```python
from build123d import *

# Parameters (mm, degrees)
F0_R      = 6.35
F1_DEPTH  = 0.254
F2_R      = 3.429
F3_DEPTH  = 1.905
F3_TAPER  = 20
F4_T      = 0.254
F5_R      = 1.0795
F6_DEPTH  = 25.4
F7_R      = 0.3175
F8_DEPTH  = 25.4
F9_R      = 0.3175
F10_DEPTH = 25.4


# Not quite as in the source:
# - a shell that OpenCascade refuses in one call is made with other operations: the cavity is built on its own and cut out


with BuildPart() as f1:
    # F0 (on Top) → F1 (new body)
    with BuildSketch(Plane.XY):
        Circle(F0_R)
    extrude(amount=F1_DEPTH)

    # F2 (on face) → F3 (join)
    with BuildSketch(Plane.XY.offset(0.254)):
        Circle(F2_R)
    extrude(amount=F3_DEPTH, taper=F3_TAPER)

    # F4: shell of thickness 0.254, made by hand


with BuildPart() as f4_core1:
    # F4_t2: copy of F1
    add(f1.part)

    # the walls: a layer under each face that stays
    f4_faces = [f4_core1.faces().sort_by_distance(p)[0] for p in [
        (-6.35, 0, 0.127),
        (-4.2333333333, -4.2333333333, 0.254),
        (-3.0823183519, 0, 1.2065),
        (0, 0, 2.159),
    ]]
    thicken(f4_faces, amount=-F4_T, mode=Mode.SUBTRACT)

    # F4_s3 → F4_t4 (revolve, cut)
    with BuildSketch(Plane.XZ):
        Polygon((3.4313868193, 0.2574087312), (3.429, 0), (3.2511472853, 0), (3.1903180743, 0.1671268836), align=None)
    revolve(axis=Axis((0, 0, 0.254), (0, 0, -1)), mode=Mode.SUBTRACT)


with BuildPart() as f1_1:
    add(f1.part)

    # what is left inside the walls is the cavity
    f4_cavity = [f4_core1.part.solids().sort_by_distance(p)[0] for p in [
        (-2.977087, 0, 0.745549),
    ]]
    add(f4_cavity, mode=Mode.SUBTRACT)

    # F5 (on face) → F6 (cut)
    with BuildSketch(Plane.XY.offset(2.159)):
        Circle(F5_R)
    extrude(amount=-F6_DEPTH, mode=Mode.SUBTRACT)

    # F7 (on face) → F8 (cut)
    with BuildSketch(Plane.XY.offset(2.159)):
        with Locations((-1.3804862777, 1.0167437666)):
            Circle(F7_R)
        with Locations((-1.5707690699, -0.6871643028)):
            Circle(F7_R)
        with Locations((-0.1902827922, -1.7039080694)):
            Circle(F7_R)
        with Locations((1.3804862777, -1.0167437666)):
            Circle(F7_R)
        with Locations((1.5707690699, 0.6871643028)):
            Circle(F7_R)
        with Locations((0.1902827922, 1.7039080694)):
            Circle(F7_R)
    extrude(amount=-F8_DEPTH, mode=Mode.SUBTRACT)

    # F9 (on face) → F10 (cut)
    with BuildSketch(Plane.XY.offset(0.254)):
        with Locations((-3.3923081987, 4.5992901719)):
            Circle(F9_R)
        with Locations((-5.1411364532, 2.4959849698)):
            Circle(F9_R)
        with Locations((-5.7121923037, -0.179120309)):
            Circle(F9_R)
        with Locations((-4.9746537368, -2.8131912837)):
            Circle(F9_R)
        with Locations((-3.0974819499, -4.8027940378)):
            Circle(F9_R)
        with Locations((-0.510714377, -5.6921345579)):
            Circle(F9_R)
        with Locations((2.193051705, -5.2774756484)):
            Circle(F9_R)
        with Locations((4.3944160704, -3.6538106683)):
            Circle(F9_R)
        with Locations((5.5890726726, -1.1931016973)):
            Circle(F9_R)
        with Locations((5.5033400811, 1.5409324941)):
            Circle(F9_R)
        with Locations((4.1568585995, 3.9219576214)):
            Circle(F9_R)
        with Locations((1.8580909083, 5.4045095223)):
            Circle(F9_R)
        with Locations((-0.8663430176, 5.6489534231)):
            Circle(F9_R)
    extrude(amount=-F10_DEPTH, mode=Mode.SUBTRACT)


solid = f1_1.part
```
Source: CAD feature listing. Evaluate the final solid. Frame: model axes, mm. A direction names the side the tool comes from. Give positions to 0.01 mm unless a question says otherwise; leave off trailing zeros. Order: outer loops, then holes, each group sorted by start corner. A loop starts at its lowest first (then second) coordinate and runs counter-clockwise, first axis right, second up. Notation, with made-up numbers: (-10, -19) -> (0, -19) arc R20 ccw to (0, -12) -> close; hole circle Ø3 at (-9.75, -4.75). An arc over 180 degrees is marked (long way). Use a Markdown table: item, result.
Q1. Section A-A (z = 0.8). Return the cut outline in (x, y), and give its area (3 significant figures).
A:
| item | result |
|---|---|
| outline | circle Ø6.46 at (0, 0); hole circle Ø5.92 at (0, 0) |
| area | 5.26 mm^2 |
Q2. First-contact query: P1, Ø1, axis at x = -1.5, z = 2, coming from the +Y side; P2, Ø1, axis at x = -2, y = -4.5, coming from the +Z side; P3, Ø4, axis at x = 1, y = 1, coming from the -Z side; P4, Ø2.5, axis at x = 0, y = 0, coming from the -Z side (3 decimals). Flat tips, straight axial feed; report the tip coordinate or a pass-through.
A:
| item | result |
|---|---|
| P1 | y = 2.69 |
| P2 | z = 0.25 |
| P3 | z = 0 |
| P4 | z = 1.905 |
Q3. Section B-B (x = -4.25). Return the cut outline in (y, z).
A:
| item | result |
|---|---|
| outline | (-4.72, 0) -> (4.72, 0) -> (4.72, 0.25) -> (-4.72, 0.25) -> close |
Q4. Access query for faces 1 (the face through (3, -3, 0.254)), 2 (the face through (-3, 2, 0)). Directions: +Z, -Z, +X, -X, +Y, -Y. A direction counts if a zero-diameter tool reaches every point of the face in a straight line with its end or side. Return the directions, or none.
A:
| item | result |
|---|---|
| face 1 | +Z |
| face 2 | -Z, +X, -X, +Y, -Y |
Q5. Section C-C (z = 1.6). Return the cut outline in (x, y).
A:
| item | result |
|---|---|
| outline | circle Ø5.88 at (0, 0); hole circle Ø5.34 at (0, 0) |
Q6. Material intervals for line 1 (X direction, y = 1.75, z = 0.1); line 2 (Y direction, x = -1, z = 0.3); line 3 (X direction, y = 0, z = 0.85), sorted ascending. Write a range as [from, to].
A:
| item | result |
|---|---|
| line 1 | [-6.1, -2.7], [2.7, 5.26], [5.74, 6.1] |
| line 2 | [-3.26, -2.98], [2.98, 3.26] |
| line 3 | [-3.21, -2.94], [2.94, 3.21] |
